from build123d import *

# Parameters (mm, degrees)
SKETCH_1_R      = 6
SKETCH_1_R_2    = 2.5
EXTRUDE_1_DEPTH = 3
EXTRUDE_START   = 3
SKETCH_1_3_R    = 6
SKETCH_1_3_R_2  = 2.5
EXTRUDE_2_DEPTH = 3


with BuildPart() as part:
    # 草图1 → 凸台-拉伸1 (new body)
    # profile 1 of 4: a face of its own
    with BuildSketch(Plane.XY):
        with BuildLine():
            ThreePointArc((40.464305263, 74.956398411), (33.181387998, 69.095159353), (29.012930833, 77.462893339))
            Line((29.012930833, 77.462893339), (-5.45137443, 2.506494928))
            ThreePointArc((-5.45137443, 2.506494928), (1.282917266, 5.861239058), (6, 0))
            ThreePointArc((6, 0), (4.685854424, -3.747368186), (1.319077226, -5.853207264))
            Line((1.319077226, -5.853207264), (103.75020434, 17.230644193))
            ThreePointArc((103.75020434, 17.230644193), (96.5694233, 24.364643554), (106.071305848, 27.85345299))
            Line((106.071305848, 27.85345299), (38.104483997, 79.725999944))
            ThreePointArc((38.104483997, 79.725999944), (39.842086981, 77.61712459), (40.464305263, 74.956398411))
        make_face()
    # profile 2 of 4: a face of its own
    with BuildSketch(Plane.XY):
        with Locations((34.464305263, 74.956398411)):
            Circle(SKETCH_1_R)
        with Locations((34.464305263, 74.956398411)):
            Circle(SKETCH_1_R_2, mode=Mode.SUBTRACT)
    # profile 3 of 4: a face of its own
    with BuildSketch(Plane.XY):
        Circle(SKETCH_1_R)
        Circle(SKETCH_1_R_2, mode=Mode.SUBTRACT)
    # profile 4 of 4: a face of its own
    with BuildSketch(Plane.XY):
        with Locations((102.431127114, 23.083851457)):
            Circle(SKETCH_1_R)
        with Locations((102.431127114, 23.083851457)):
            Circle(SKETCH_1_R_2, mode=Mode.SUBTRACT)
    extrude(amount=EXTRUDE_1_DEPTH)

    # 草图1<3> → 凸台-拉伸2 (add)
    with BuildSketch(Plane.XY.offset(EXTRUDE_START)):
        with Locations(Location((34.464305263, 74.956398411, 0), (0, 0, 155.307436438))):
            Circle(SKETCH_1_3_R)
        with Locations((34.464305263, 74.956398411)):
            Circle(SKETCH_1_3_R_2, mode=Mode.SUBTRACT)
    extrude(amount=EXTRUDE_2_DEPTH)


solid = part.part
Can you work these out from the model? Positions are in its coordinate system, mm. Round coordinates to 2 decimals unless told otherwise and drop trailing zeros. Loops run counter-clockwise (first coordinate to the right, second up) from the corner with the lowest first, then second, coordinate; pieces in that order, holes last. Notation, with made-up numbers: (44.5, -11) - (84.5, -11) arc R30 ccw to (84.5, 20) - close; hole circle Ø7 at (86.25, 77.25). An arc over 180 degrees is marked (long way). Answer in a Markdown table with one row per item. Add a question column.
Q1. I want a section at A-A on y = 0. List the corners of the cut face in (x, z) for me, and give its area (3 significant figures).
Q2. I want a section at B-B on x = 0. List the corners of the cut face in (y, z) for me.
Q3. I want a section at C-C on z = 1.6. List the corners of the cut face in (x, y) for me.
Q4. I need wall thicknesses on L1, parallel to X at y = 75, z = 4.7; L2, parallel to Z at x = 45, y = 21; L3, parallel to Y at x = 0, z = 1.15. Which ranges of each line are inside material? Lowest first, please.
Q5. I want a section at D-D on x = 58.5. List the corners of the cut face in (y, z) for me, and give its area (3 significant figures).
Q6. For pin 1 Ø8 at (x, y) = (47, 62.5) entering from +Z; pin 2 Ø3 at (x, y) = (34.46, 74.96) entering from -Z; pin 3 Ø1.5 at (x, z) = (25, 3) entering from -Y, each with a flat end and sliding along its axis, tell me the tip position at first contact or that it passes through.
Q7. We'd pull the mould along X, two halves only. Please class faces 1 (the cylindrical face through (-0.54, -2.44, 1.48)), 2 (the cylindrical face through (36.006, 80.755, 2.958)), 3 (the cylindrical face through (108.27, 21.71, 1.48)): pulls with the +X half, pulls with the -X half, needs draft (parallel to the pull), parting line crosses it, or undercut.
A:
| question | item | result |
|---|---|---|
| 1 | outline | (-6, 0) - (-2.5, 0) - (-2.5, 3) - (-6, 3) - close; (2.5, 0) - (27.29, 0) - (27.29, 3) - (2.5, 3) - close |
| 1 | area | 84.9 mm^2 |
| 2 | outline | (-6, 0) - (-2.5, 0) - (-2.5, 3) - (-6, 3) - close; (2.5, 0) - (14.36, 0) - (14.36, 3) - (2.5, 3) - close |
| 3 | outline | (-5.45, 2.51) arc R6 ccw to (1.32, -5.85) - (103.75, 17.23) arc R6 ccw to (106.07, 27.85) - (38.1, 79.73) arc R6 ccw to (29.01, 77.46) - close; hole circle Ø5 at (0, 0); hole circle Ø5 at (34.46, 74.96); hole circle Ø5 at (102.43, 23.08) |
| 4 | L1 | 28.46 to 31.96, 36.96 to 40.46 |
| 4 | L2 | 0 to 3 |
| 4 | L3 | -6 to -2.5, 2.5 to 14.36 |
| 5 | outline | (7.03, 0) - (64.16, 0) - (64.16, 3) - (7.03, 3) - close |
| 5 | area | 171 mm^2 |
| 6 | pin 1 | z = 3 |
| 6 | pin 2 | through |
| 6 | pin 3 | y = -0.69 |
| 7 | face 1 | undercut |
| 7 | face 2 | parting line crosses it |
| 7 | face 3 | pulls with the +X half |
